Part model, mm, in its own coordinate system. A direction names the side the tool comes from. Give positions to 0.01 mm unless a question says otherwise; leave off trailing zeros. Write each loop counter-clockwise with the first axis right and the second up, starting at its lowest first coordinate (ties: lowest second). Pieces come first, ordered by that corner, then holes. Notation, with made-up numbers: (5.5, 65.25) - (47.5, 65.25) arc R31 cw to (47.5, 89.25) - close; hole circle Ø10 at (7.25, 42.25). An arc over 180 degrees is marked (long way). Answer in a Markdown table with one row per item. Add a question column.
1. Band-saw the part on B-B on y = -20. Write the cut outline in (x, z).
2. Drop flat-ended pins along their axis: pin 1 Ø3.5 at (x, z) = (-18.37, 14.98) entering from +Y; pin 2 Ø3 at (y, z) = (-8.5, 10) entering from +X; pin 3 Ø10 at (y, z) = (-22.5, 6) entering from +X; pin 4 Ø6 at (x, z) = (-19, 9.5) entering from +Y. Give the stop position or say it passes through.
3. Band-saw the part on A-A on x = -17. Write the cut outline in (y, z), plus the area to 3 significant figures.
4. Which spindle directions (+Z, -Z, +X, -X, +Y, -Y) get a long thin tool onto all of the face, cutting with end or side? Do faces 5 (the flat face through (-17, -9, 1.45)), 6 (the flat face through (27, -11.825, 10)), 7 (the flat face through (30, -11, 16.775)), 8 (the flat face through (-21, -11, 13.175)). Say none if no direction does.
5. Probe line 1 along X through (y, z) = (-27.5, 9); line 2 along Y through (x, z) = (18, 18.5); line 3 along Y through (x, z) = (-15.5, 10.25). List the from-to ranges inside material, lowest first.
6. Pull direction Z, two halves, no side cores. Call faces 1 (the flat face through (27, -9, 18.5)), 2 (the flat face through (4, -25, 0)), 3 (the flat face through (4, -44.125, 10)), 4 (the flat face through (4, -25, 19.95)): released by +Z, released by -Z, zero draft, split by the parting line, or undercut.
```python
from build123d import *

# Parameters (mm, degrees)
EXTRUDE_1_DEPTH     = 19.95
SKETCH_2_W          = 7.4
SKETCH_2_H          = 1.45
EXTRUDE_2_DEPTH     = 1.45
CHAMFER_1_SIZE      = 1.45
CHAMFER_1_SIZE2     = 2
CHAMFER_3_SIZE      = 1.45
CHAMFER_3_SIZE2     = 2
CHAMFER_4_SIZE      = 1.45
CHAMFER_4_SIZE2     = 2
CHAMFER_5_SIZE      = 1.45
CHAMFER_5_SIZE2     = 2
SKETCH_3_R          = 2.25
CUT_EXTRUDE_1_DEPTH = 2
SKETCH_4_W          = 2.602143293
SKETCH_4_H          = 3.6
SKETCH_4_W_2        = 2.852203288
CUT_EXTRUDE_2_DEPTH = 2
SKETCH_5_R          = 6.2
EXTRUDE_3_DEPTH     = 2
CHAMFER_6_SIZE      = 1
SKETCH_6_R          = 3
EXTRUDE_4_DEPTH     = 3


with BuildPart() as part:
    # 草圖1 → 填料-伸長1 (new body)
    with BuildSketch(Plane.XY):
        Polygon((-14.470198675, -11.825165563), (-14.470198675, -44.125165563), (23.929801325, -44.125165563), (23.929801325, -11.825165563), (31.329801325, -11.825165563), (31.329801325, -9.825165563), (23.929801325, -9.825165563), (23.929801325, -6.325165563), (-14.470198675, -6.325165563), (-14.470198675, -9.825165563), (-21.870198675, -9.825165563), (-21.870198675, -11.825165563), align=None)
    extrude(amount=EXTRUDE_1_DEPTH)

    # 草圖2 → 填料-伸長2 (add)
    with BuildSketch(Plane(origin=(0, -9.825165563, 0), x_dir=(1, 0, 0), z_dir=(0, 1, 0))):
        with Locations((27.629801325, -0.725)):
            Rectangle(SKETCH_2_W, SKETCH_2_H)
        with Locations((27.629801325, -19.225)):
            Rectangle(SKETCH_2_W, SKETCH_2_H)
        with Locations((-18.170198675, -0.725)):
            Rectangle(SKETCH_2_W, SKETCH_2_H)
        with Locations((-18.170198675, -19.225)):
            Rectangle(SKETCH_2_W, SKETCH_2_H)
    extrude(amount=EXTRUDE_2_DEPTH)

    # 導角1
    chamfer_1_edges = [part.edges().sort_by_distance(p)[0] for p in [
        (31.329801325, -8.375165563, 19.225),
    ]]
    chamfer_1_side = [part.faces().sort_by_distance(p)[0] for p in [
        (31.329801325, -10.660702917, 9.975),
    ]]
    chamfer(chamfer_1_edges, length=CHAMFER_1_SIZE, length2=CHAMFER_1_SIZE2, reference=chamfer_1_side[0])

    # 導角3
    chamfer_3_edges = [part.edges().sort_by_distance(p)[0] for p in [
        (31.329801325, -8.375165563, 0.725),
    ]]
    chamfer_3_side = [part.faces().sort_by_distance(p)[0] for p in [
        (31.329801325, -10.738818024, 9.511976966),
    ]]
    chamfer(chamfer_3_edges, length=CHAMFER_3_SIZE, length2=CHAMFER_3_SIZE2, reference=chamfer_3_side[0])

    # 導角4
    chamfer_4_edges = [part.edges().sort_by_distance(p)[0] for p in [
        (-21.870198675, -8.375165563, 19.225),
    ]]
    chamfer_4_side = [part.faces().sort_by_distance(p)[0] for p in [
        (-21.870198675, -10.660702917, 9.975),
    ]]
    chamfer(chamfer_4_edges, length=CHAMFER_4_SIZE, length2=CHAMFER_4_SIZE2, reference=chamfer_4_side[0])

    # 導角5
    chamfer_5_edges = [part.edges().sort_by_distance(p)[0] for p in [
        (-21.870198675, -8.375165563, 0.725),
    ]]
    chamfer_5_side = [part.faces().sort_by_distance(p)[0] for p in [
        (-21.870198675, -10.738818024, 9.511976966),
    ]]
    chamfer(chamfer_5_edges, length=CHAMFER_5_SIZE, length2=CHAMFER_5_SIZE2, reference=chamfer_5_side[0])

    # 草圖3 → 除料-伸長1 (cut)
    with BuildSketch(Plane(origin=(0, -9.825165563, 0), x_dir=(1, 0, 0), z_dir=(0, 1, 0))):
        with Locations(Location((-18.370198675, -4.975, 0), (0, 0, 180))):
            Circle(SKETCH_3_R)
        with Locations(Location((-18.370198675, -14.975, 0), (0, 0, 180))):
            Circle(SKETCH_3_R)
        with Locations(Location((27.829801325, -14.975, 0), (0, 0, 180))):
            Circle(SKETCH_3_R)
        with Locations(Location((27.829801325, -4.975, 0), (0, 0, 180))):
            Circle(SKETCH_3_R)
    extrude(amount=-CUT_EXTRUDE_1_DEPTH, mode=Mode.SUBTRACT)

    # 草圖4 → 除料-伸長2 (cut)
    with BuildSketch(Plane(origin=(0, -9.825165563, 0), x_dir=(1, 0, 0), z_dir=(0, 1, 0))):
        with Locations((-20.569127028, -14.975)):
            Rectangle(SKETCH_4_W, SKETCH_4_H)
        with Locations((-20.569127028, -4.975)):
            Rectangle(SKETCH_4_W, SKETCH_4_H)
        with Locations((29.903699681, -14.975)):
            Rectangle(SKETCH_4_W_2, SKETCH_4_H)
        with Locations((29.903699681, -4.975)):
            Rectangle(SKETCH_4_W_2, SKETCH_4_H)
    extrude(amount=-CUT_EXTRUDE_2_DEPTH, mode=Mode.SUBTRACT)

    # 草圖5 → 填料-伸長3 (add)
    with BuildSketch(Plane(origin=(0, -6.325165563, 0), x_dir=(1, 0, 0), z_dir=(0, 1, 0))):
        with Locations((14.349801325, -9.975)):
            Circle(SKETCH_5_R)
    extrude(amount=EXTRUDE_3_DEPTH)

    # 導角6
    chamfer_6_edges = [part.edges().sort_by_distance(p)[0] for p in [
        (8.149801325, -4.325165563, 9.975),
    ]]
    chamfer(chamfer_6_edges, length=CHAMFER_6_SIZE)

    # 草圖6 → 填料-伸長4 (add)
    with BuildSketch(Plane(origin=(0, -4.325165563, 0), x_dir=(1, 0, 0), z_dir=(0, 1, 0))):
        with Locations(Location((14.349801325, -9.975, 0), (0, 0, 180))):
            Circle(SKETCH_6_R)
    extrude(amount=EXTRUDE_4_DEPTH)


solid = part.part
```
Values:
| question | item | result |
|---|---|---|
| 1 | outline | (-14.47, 0) - (23.93, 0) - (23.93, 19.95) - (-14.47, 19.95) - close |
| 2 | pin 1 | passes through |
| 2 | pin 2 | stops at x = 31.33 |
| 2 | pin 3 | stops at x = 23.93 |
| 2 | pin 4 | stops at y = -9.83 |
| 3 | outline | (-11.83, 0) - (-8.38, 0) - (-8.38, 1.45) - (-9.83, 1.45) - (-9.83, 3.19) - (-11.83, 3.19) - close; (-11.83, 6.76) - (-9.83, 6.76) - (-9.83, 13.19) - (-11.83, 13.19) - close; (-11.83, 16.76) - (-9.83, 16.76) - (-9.83, 18.5) - (-8.38, 18.5) - (-8.38, 19.95) - (-11.83, 19.95) - close |
| 3 | area | 29.8 mm² |
| 4 | face 5 | -X, +Y |
| 4 | face 6 | +Z, -Z, +X, -Y |
| 4 | face 7 | +X, +Y, -Y |
| 4 | face 8 | -X, +Y, -Y |
| 5 | line 1 | x = -14.47 to 23.93 |
| 5 | line 2 | y = -44.13 to -6.33 |
| 5 | line 3 | y = -11.83 to -9.83 |
| 6 | face 1 | undercut |
| 6 | face 2 | released by -Z |
| 6 | face 3 | zero draft |
| 6 | face 4 | released by +Z |
